from build123d import *

# Parameters (mm, degrees)
SKETCH_1_W               = 10
SKETCH_1_H               = 38
SKETCH_1_R               = 1.1
EXTRUDE_1_DEPTH          = 0.75
EXTRUDE_1_DEPTH_BACK     = 0.75
SKETCH_3_W               = 20
SKETCH_3_H               = 38.036879249
EXTRUDE_2_DEPTH          = 1.5
EXTRUDE_3_DEPTH          = 1
EXTRUDE_3_DEPTH_BACK     = 1
EXTRUDE_4_DEPTH          = 38
CUT_EXTRUDE_1_DEPTH      = 10
CUT_EXTRUDE_1_DEPTH_BACK = 20
SKETCH_10_W              = 112.497058814
SKETCH_10_H              = 20.543414641
CUT_EXTRUDE_4_DEPTH      = 0.2
CUT_EXTRUDE_4_DEPTH_BACK = 0.2
SKETCH_11_W              = 104.514605189
SKETCH_11_H              = 21.657747512
CUT_EXTRUDE_5_DEPTH      = 0.2
CUT_EXTRUDE_5_DEPTH_BACK = 0.2


with BuildPart() as part:
    # Sketch 1 → Extrude 1 (new body, two sides)
    with BuildSketch(Plane.XY) as extrude_1_sk:
        with Locations((-4.101832994, 0.735234216)):
            Rectangle(SKETCH_1_W, SKETCH_1_H)
        with Locations((-6.601832994, -15.764765784)):
            Circle(SKETCH_1_R, mode=Mode.SUBTRACT)
        with Locations((-6.578411405, 17.235234216)):
            Circle(SKETCH_1_R, mode=Mode.SUBTRACT)
    extrude(amount=EXTRUDE_1_DEPTH)
    extrude(extrude_1_sk.sketch, amount=-EXTRUDE_1_DEPTH_BACK)

    # Sketch 3 → Extrude 2 (add)
    with BuildSketch(Plane(origin=(-0.5, 0, 0), x_dir=(0, 0, -1), z_dir=(1, 0, 0))):
        with Locations((0, 0.716794592)):
            Rectangle(SKETCH_3_W, SKETCH_3_H)
    extrude(amount=EXTRUDE_2_DEPTH)

    # Sketch 4 → Extrude 3 (add, two sides)
    with BuildSketch(Plane.XY) as extrude_3_sk:
        with BuildLine():
            Line((1, 19.735234216), (1, -18.298860138))
            ThreePointArc((1, -18.298860138), (51.989546932, -13.993809638), (101, 0.718187039))
            ThreePointArc((101, 0.718187039), (51.989546932, 15.430183716), (1, 19.735234216))
        make_face()
    extrude(amount=EXTRUDE_3_DEPTH)
    extrude(extrude_3_sk.sketch, amount=-EXTRUDE_3_DEPTH_BACK)

    # Sketch 5 → Extrude 4 (add)
    with BuildSketch(Plane(origin=(0, 19.735234216, 0), x_dir=(1, 0, 0), z_dir=(0, 1, 0))):
        with BuildLine():
            Line((1, -8), (1, -10))
            ThreePointArc((1, -10), (50.655745388, -8.426256946), (100.20651497, -4.835859882))
            Line((100.20651497, -4.835859882), (100.20651497, -2.835859882))
            ThreePointArc((100.20651497, -2.835859882), (50.661805416, -6.542674054), (1, -8))
        make_face()
        with BuildLine():
            Line((100.20651497, 2.835859882), (100.20651497, 4.835859882))
            ThreePointArc((100.20651497, 4.835859882), (50.655745388, 8.426256946), (1, 10))
            Line((1, 10), (1, 8))
            ThreePointArc((1, 8), (50.661805416, 6.542674054), (100.20651497, 2.835859882))
        make_face()
    extrude(amount=-EXTRUDE_4_DEPTH)

    # Sketch 8 → Cut-Extrude 1 (cut, two sides)
    with BuildSketch(Plane.XY.offset(10)) as cut_extrude_1_sk:
        with BuildLine():
            Line((13.103688801, -18.23809131), (101, -18.264765784))
            Line((101, -18.264765784), (101, 0.718187039))
            ThreePointArc((101, 0.718187039), (57.921072507, -12.790381672), (13.103688801, -18.23809131))
        make_face()
        with BuildLine():
            ThreePointArc((13.103688801, 19.674465387), (57.921072507, 14.22675575), (101, 0.718187039))
            Line((101, 0.718187039), (101, 19.701139862))
            Line((101, 19.701139862), (13.103688801, 19.674465387))
        make_face()
    extrude(amount=CUT_EXTRUDE_1_DEPTH, mode=Mode.SUBTRACT)
    extrude(cut_extrude_1_sk.sketch, amount=-CUT_EXTRUDE_1_DEPTH_BACK, mode=Mode.SUBTRACT)

    # Sketch 10 → Cut-Extrude 4 (cut, two sides)
    with BuildSketch(Plane(origin=(0, 19.735234216, 0), x_dir=(1, 0, 0), z_dir=(0, 1, 0))) as cut_extrude_4_sk:
        with Locations((46.49437126, 0.271707321)):
            Rectangle(SKETCH_10_W, SKETCH_10_H)
    extrude(amount=CUT_EXTRUDE_4_DEPTH, mode=Mode.SUBTRACT)
    extrude(cut_extrude_4_sk.sketch, amount=-CUT_EXTRUDE_4_DEPTH_BACK, mode=Mode.SUBTRACT)

    # Sketch 11 → Cut-Extrude 5 (cut, two sides)
    with BuildSketch(Plane(origin=(0, -18.301645033, 0), x_dir=(-1, 0, 0), z_dir=(0, -1, 0))) as cut_extrude_5_sk:
        with Locations((-51.541283716, 0.828873756)):
            Rectangle(SKETCH_11_W, SKETCH_11_H)
    extrude(amount=CUT_EXTRUDE_5_DEPTH, mode=Mode.SUBTRACT)
    extrude(cut_extrude_5_sk.sketch, amount=-CUT_EXTRUDE_5_DEPTH_BACK, mode=Mode.SUBTRACT)


solid = part.part
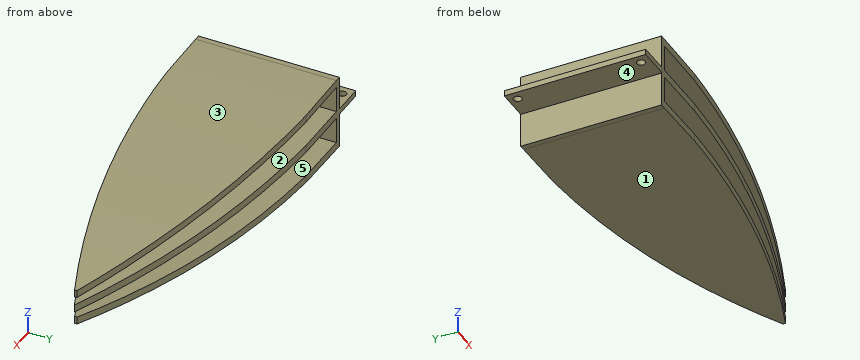
Here's how the part is built. I have some questions about the finished solid (model axes, mm). Face numbers are marked on the shaded views. A direction names the side the tool comes from. Round coordinates to 2 decimals unless told otherwise and drop trailing zeros. Write each loop counter-clockwise with the first axis right and the second up, starting at its lowest first coordinate (ties: lowest second). Pieces come first, ordered by that corner, then holes.
1. Will these pins go through, and if not, where does the flat tip stop? pin 1 Ø0.5 at (y, z) = (0.5, 3.5) entering from +X; pin 2 Ø12 at (x, z) = (79, 7) entering from -Y; pin 3 Ø11.5 at (x, y) = (44, 2.5) entering from -Z.
2. If we mould it in two halves opening along Z, with no side actions, what happens to the marked faces 1, 2 and 3? For each: released by +Z, released by -Z, zero draft, split by the parting line, or undercut.
3. Suppose I cut it at B-B (z = 6.25). List the corners of the cut face in (x, y) for me.
4. For the marked faces 4 and 5, which set-ups out of +Z, -Z, +X, -X, +Y, -Y let a thin tool reach every point of the face, with its end or its side?
5. I need wall thicknesses on L1, parallel to Z at x = 45.5, y = -7.5; L2, parallel to Z at x = 18.5, y = -1; L3, parallel to X at y = -3, z = -2.75. Which ranges of each line are inside material? Lowest first, please.
6. Suppose I cut it at D-D (x = 70). List the corners of the cut face in (y, z) for me.
7. Suppose I cut it at C-C (y = 10). List the corners of the cut face in (x, z) for me, and give its area (3 significant figures).
8. Suppose I cut it at A-A (x = 55.5). List the corners of the cut face in (y, z) for me.
Answer sheet:
1. pin 1: stops at x = 100.21
1. pin 2: stops at y = -9.04
1. pin 3: stops at z = -9.01
2. face 1: released by -Z
2. face 2: undercut
2. face 3: released by +Z
3. outline: (-0.5, -18.1) - (1, -18.1) - (1, 19.54) - (-0.5, 19.54) - close; (56.03, -13.19) arc R247.18 ccw to (83.79, -5.72) - (83.79, 7.16) arc R247.18 ccw to (56.03, 14.63) - close
4. face 4: -Z, -X, +Y, -Y
4. face 5: +Y, -Y
5. L1: z = -8.68 to -6.8, -1 to 1, 6.8 to 8.68
5. L2: z = -9.68 to -7.74, -1 to 1, 7.74 to 9.68
5. L3: x = -0.5 to 1
6. outline: (-9.87, -7.27) - (11.3, -7.27) - (11.3, -5.36) - (-9.87, -5.36) - close; (-9.87, -1) - (11.3, -1) - (11.3, 1) - (-9.87, 1) - close; (-9.87, 5.36) - (11.3, 5.36) - (11.3, 7.27) - (-9.87, 7.27) - close
7. outline: (-9.1, -0.75) - (-0.5, -0.75) - (-0.5, -10) - (1, -10) arc R1222.24 ccw to (74.66, -6.94) - (74.66, -5.03) arc R1095.84 cw to (1, -8) - (1, -1) - (74.66, -1) - (74.66, 1) - (1, 1) - (1, 8) arc R1095.84 cw to (74.66, 5.03) - (74.66, 6.94) arc R1222.24 ccw to (1, 10) - (-0.5, 10) - (-0.5, 0.75) - (-9.1, 0.75) - close
7. area: 472 mm2
8. outline: (-13.3, -8.16) - (14.74, -8.16) - (14.74, -6.28) - (-13.3, -6.28) - close; (-13.3, -1) - (14.74, -1) - (14.74, 1) - (-13.3, 1) - close; (-13.3, 6.28) - (14.74, 6.28) - (14.74, 8.16) - (-13.3, 8.16) - close
